Read the model definition and answer for the solid it produces. Units are mm, in the model's axes. Coordinates: 2 decimals unless noted, no trailing zeros. Loops run counter-clockwise (first coordinate to the right, second up) from the corner with the lowest first, then second, coordinate; pieces in that order, holes last. Notation, with made-up numbers: M 54.25,77 L 79.25,77 A8 ccw 79.25,91 Z; hole C -26.75,19 d7. An arc over 180 degrees is marked long. Use one line per item in the form item = value. Start each with the question number.
1. Find the intervals of material crossed by probe 1 along Y at (x, z) = (-1.75, 0); probe 2 along X at (y, z) = (7.5, -0.05); probe 3 along Y at (x, z) = (-0.9, -1.2), in increasing order. Write a range as [from, to].
2. Flat-ended cylindrical pins translate along their axes: pin 1 (2 mm diameter, centred on x = 1.5, y = 10.5, fed in from +Z); pin 2 (2 mm diameter, centred on x = -1.5, z = -1.5, fed in from +Y); pin 3 (0.6 mm diameter, centred on y = 13.5, z = 1.5, fed in from +X). Find the tip coordinate at first contact, or state that the pin passes through.
3. The part is cut by section B-B (x = 0). Give the vertices of the cut face in (y, z), plus the area to 3 significant figures.
4. The part is cut by section C-C (y = 15). Give the number of separate pieces and of enclosed holes in the cut face, plus the area to 3 significant figures.
5. The part is cut by section A-A (y = 10.25). Give the vertices of the cut face in (x, z), plus the area to 3 significant figures.
6. For a pull along Y with two mould halves and no side action, classify faces 1 (the cylindrical face through (-0.06, 1.88, 1.46)), 2 (the flat face through (0, 7.24, -2)), 3 (the cylindrical face through (-2, 15, -0.5)), 4 (the cylindrical face through (1.96, 15.444, 0.231)) as released by +Y, released by -Y, zero draft, split by the parting line, or undercut.
from build123d import *

# Parameters (mm, degrees)
SKETCH1_R               = 2.15
BOSS_EXTRUDE1_DEPTH     = 3.12
SKETCH2_R               = 2.35
BOSS_EXTRUDE2_DEPTH     = 14.2
SHELL1_T                = -0.69
CUT_EXTRUDE2_DEPTH      = 10
CUT_EXTRUDE2_DEPTH_BACK = 10
SKETCH9_W               = 1.46
SKETCH9_H               = 4.728587073
CUT_EXTRUDE3_DEPTH      = 10.08
CUT_EXTRUDE4_DEPTH      = 10.08
CUT_EXTRUDE4_DEPTH_BACK = 10.08
SKETCH11_R              = 0.5


with BuildPart() as part:
    # Sketch1 → Boss-Extrude1 (new body)
    with BuildSketch(Plane(origin=(0, 0, 0), x_dir=(1, 0, 0), z_dir=(0, 1, 0))):
        with Locations(Location((0, 0, 0), (0, 0, 90))):
            Circle(SKETCH1_R)
    extrude(amount=BOSS_EXTRUDE1_DEPTH)

    # Sketch2 → Boss-Extrude2 (add)
    with BuildSketch(Plane(origin=(0, 3.12, 0), x_dir=(1, 0, 0), z_dir=(0, 1, 0))):
        with Locations(Location((0, 0, 0), (0, 0, 270))):
            Circle(SKETCH2_R)
    extrude(amount=BOSS_EXTRUDE2_DEPTH)

    # Shell1
    shell1_openings = [part.faces().sort_by_distance(p)[0] for p in [
        (0, 0, 0),
        (0, 17.32, 0),
    ]]
    offset(amount=SHELL1_T, openings=shell1_openings, kind=Kind.INTERSECTION)

    # Sketch7 → Cut-Extrude2 (cut, two sides: drawn at the far end of the back side and taken through both)
    with BuildSketch(Plane(origin=(0, 0, 0), x_dir=(0, 0, -1), z_dir=(1, 0, 0)).offset(-CUT_EXTRUDE2_DEPTH_BACK)):
        with BuildLine():
            Line((-4.35, 13.399999995), (-2.35, 13.399999995))
            add(Edge.make_bspline(
                [(2.35, 13.399999995), (2.35, 17.133503588), (0, 17.133503588), (-2.35, 17.133503588), (-2.35, 13.399999995)],
                knots=[4.71238898, 4.71238898, 4.71238898, 6.283185307, 6.283185307, 7.853981634, 7.853981634, 7.853981634], degree=2, weights=[1, 0.707106781, 1, 0.707106781, 1]))
            Line((2.35, 13.399999995), (4.35, 13.399999995))
            add(Edge.make_bspline(
                [(4.35, 13.399999995), (4.35, 14.065444098), (4.192339822, 15.412663566), (3.474819887, 17.250199614), (2.38815107, 18.531514052), (1.114988399, 19.194360722), (0, 19.382819631), (-1.114988399, 19.194360722), (-2.38815107, 18.531514052), (-3.474819887, 17.250199614), (-4.192339822, 15.412663566), (-4.35, 14.065444098), (-4.35, 13.399999995)],
                knots=[-1.570796327, -1.570796327, -1.570796327, -1.570796327, -1.178097245, -0.785398163, -0.392699082, -0.196349541, 0, 0.196349541, 0.392699082, 0.785398163, 1.178097245, 1.570796327, 1.570796327, 1.570796327, 1.570796327], degree=3))
        make_face()
    extrude(amount=CUT_EXTRUDE2_DEPTH + CUT_EXTRUDE2_DEPTH_BACK, mode=Mode.SUBTRACT)

    # Sketch9 → Cut-Extrude3 (cut)
    with BuildSketch(Plane(origin=(0, 17.32, 0), x_dir=(-1, 0, 0), z_dir=(0, -1, 0))):
        with Locations((0, -0.000375881)):
            Rectangle(SKETCH9_W, SKETCH9_H)
    extrude(amount=CUT_EXTRUDE3_DEPTH, mode=Mode.SUBTRACT)

    # Sketch11 → Cut-Extrude4 (cut, two sides: drawn at the far end of the back side and taken through both)
    with BuildSketch(Plane(origin=(0, 0, 0), x_dir=(0, 0, -1), z_dir=(1, 0, 0)).offset(-CUT_EXTRUDE4_DEPTH_BACK)):
        with Locations(Location((0, 15, 0), (0, 0, 180))):
            Circle(SKETCH11_R)
    extrude(amount=CUT_EXTRUDE4_DEPTH + CUT_EXTRUDE4_DEPTH_BACK, mode=Mode.SUBTRACT)


solid = part.part
Computed values:
q1.probe_1 = [0, 14.5], [15.5, 17.13]
q1.probe_2 = [-2.35, -1.66], [1.66, 2.35]
q1.probe_3 = [0, 3.81]
q2.pin_1 = 2.23
q2.pin_2 = 17.05
q2.pin_3 = 2.02
q3.outline = M 0,-2.15 L 3.12,-2.15 L 3.12,-2.35 L 7.24,-2.35 L 7.24,-1.66 L 3.81,-1.66 L 3.81,-1.46 L 0,-1.46 Z; M 0,1.46 L 3.81,1.46 L 3.81,1.66 L 7.24,1.66 L 7.24,2.35 L 3.12,2.35 L 3.12,2.15 L 0,2.15 Z
q3.area = 10.3 mm²
q4.separate_pieces = 4
q4.enclosed_holes = 0
q4.area = 5.17 mm²
q5.outline = M -0.73,-2.23 L -0.73,-1.49 A1.66 cw -0.73,1.49 L -0.73,2.23 A2.35 ccw Z; M 0.73,-2.23 A2.35 ccw 0.73,2.23 L 0.73,1.49 A1.66 cw 0.73,-1.49 Z
q5.area = 6.63 mm²
q6.face_1 = zero draft
q6.face_2 = released by +Y
q6.face_3 = undercut
q6.face_4 = undercut
